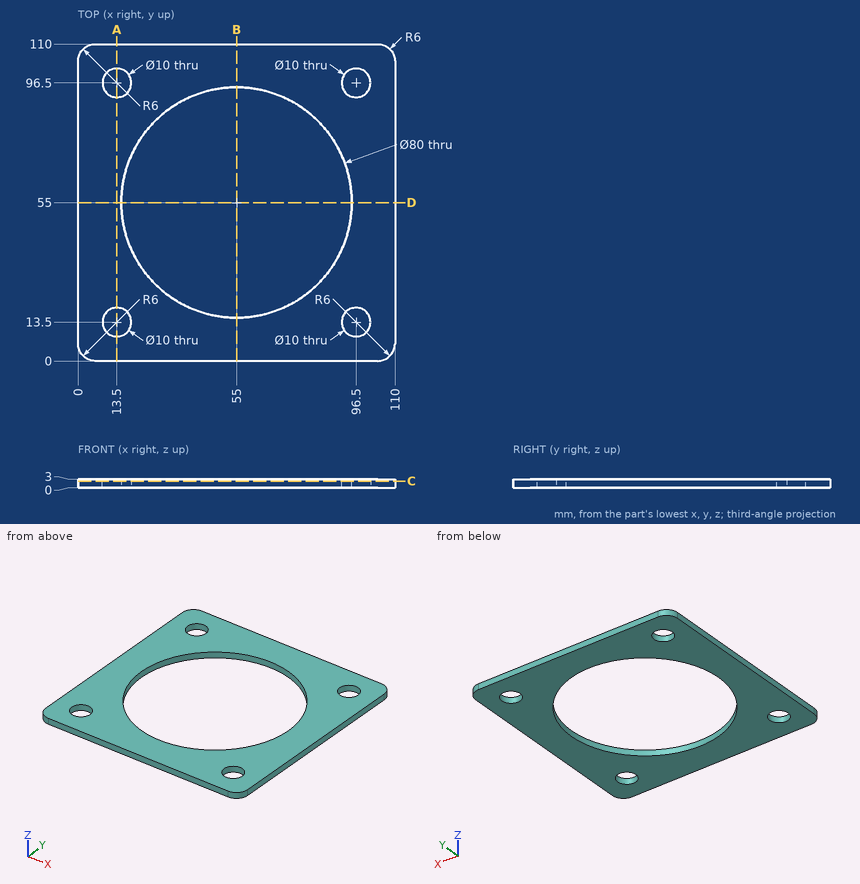
Design review of the part shown in the three views and the two pictorial views. Dimensions are in mm from the part's minimum x, y and z. Round coordinates to 2 decimals unless told otherwise and drop trailing zeros. Write each loop counter-clockwise with the first axis right and the second up, starting at its lowest first coordinate (ties: lowest second). Pieces come first, ordered by that corner, then holes.
Item 1: We need section B-B on x = 55. Write out the cut boundary in (y, z).
Item 2: We need section C-C on z = 2.25. Write out the cut boundary in (x, y), and give its area (3 significant figures).
Item 3: We need section A-A on x = 13.5. Write out the cut boundary in (y, z), and give its area (3 significant figures).
Item 4: For probe 1 along Y at (x, z) = (13.5, 1.35); probe 2 along X at (y, z) = (9, 2.35); probe 3 along X at (y, z) = (55, 1.15), list the stretches that pass through material, from the lowest coordinate up.
Returned:
1. outline: (0, 0) - (15, 0) - (15, 3) - (0, 3) - close; (95, 0) - (110, 0) - (110, 3) - (95, 3) - close
2. outline: (0, 6) arc R6 ccw to (6, 0) - (104, 0) arc R6 ccw to (110, 6) - (110, 104) arc R6 ccw to (104, 110) - (6, 110) arc R6 ccw to (0, 104) - close; hole circle Ø10 at (13.5, 13.5); hole circle Ø10 at (13.5, 96.5); hole circle Ø80 at (55, 55); hole circle Ø10 at (96.5, 13.5); hole circle Ø10 at (96.5, 96.5)
2. area: 6,730 mm2
3. outline: (0, 0) - (8.5, 0) - (8.5, 3) - (0, 3) - close; (18.5, 0) - (91.5, 0) - (91.5, 3) - (18.5, 3) - close; (101.5, 0) - (110, 0) - (110, 3) - (101.5, 3) - close
3. area: 270 mm2
4. probe 1: y = 0 to 8.5, 18.5 to 91.5, 101.5 to 110
4. probe 2: x = 0 to 11.32, 15.68 to 94.32, 98.68 to 110
4. probe 3: x = 0 to 15, 95 to 110
